from build123d import *

# Parameters (mm, degrees)
SKETCH3_W           = 76.2
SKETCH3_H           = 76.2
BOSS_EXTRUDE2_DEPTH = 101.6
SKETCH4_R           = 6.35
CUT_EXTRUDE2_DEPTH  = 73.914
SKETCH5_R           = 25.4
CUT_EXTRUDE3_DEPTH  = 113.538
SKETCH7_R           = 6.35
CUT_EXTRUDE4_DEPTH  = 18.034


with BuildPart() as part:
    # Sketch3 → Boss-Extrude2 (new body)
    with BuildSketch(Plane(origin=(0, 0, 0), x_dir=(1, 0, 0), z_dir=(0, 1, 0))):
        with Locations((38.1, 38.1)):
            Rectangle(SKETCH3_W, SKETCH3_H)
    extrude(amount=BOSS_EXTRUDE2_DEPTH)

    # Sketch4 → Cut-Extrude2 (cut)
    with BuildSketch(Plane.XY):
        with Locations((38.1, 50.8)):
            Circle(SKETCH4_R)
    extrude(amount=-CUT_EXTRUDE2_DEPTH, mode=Mode.SUBTRACT)

    # Sketch5 → Cut-Extrude3 (cut)
    with BuildSketch(Plane(origin=(0, 101.6, 0), x_dir=(1, 0, 0), z_dir=(0, 1, 0))):
        with Locations(Location((38.1, 38.1, 0), (0, 0, 270))):
            Circle(SKETCH5_R)
    extrude(amount=-CUT_EXTRUDE3_DEPTH, mode=Mode.SUBTRACT)

    # Sketch7 → Cut-Extrude4 (cut)
    with BuildSketch(Plane(origin=(0, 0, -76.2), x_dir=(-1, 0, 0), z_dir=(0, 0, -1))):
        with Locations(Location((-38.1, 50.8, 0), (0, 0, 180))):
            Circle(SKETCH7_R)
    extrude(amount=-CUT_EXTRUDE4_DEPTH, mode=Mode.SUBTRACT)


solid = part.part
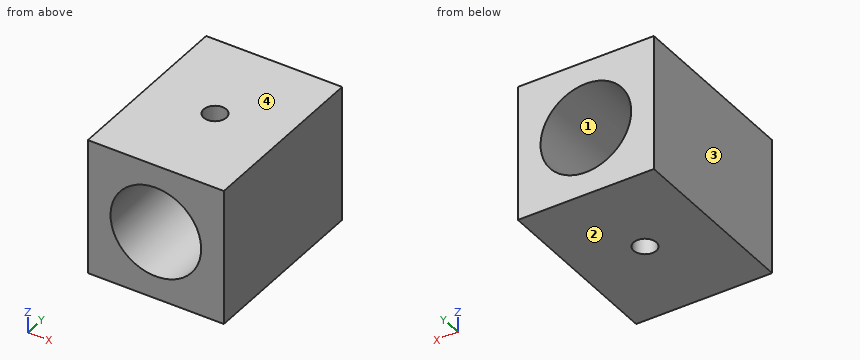
Geometry check sheet. Reference: the model listing, model coordinates, mm. Face numbers are marked on the shaded views. Give positions to 0.01 mm unless a question says otherwise; leave off trailing zeros. Write each loop counter-clockwise with the first axis right and the second up, starting at its lowest first coordinate (ties: lowest second). Pieces come first, ordered by that corner, then holes. Notation, with made-up numbers: M -8,65.5 L 33,65.5 A26 cw 33,86.5 Z; hole C -34.75,-33.75 d8. An arc over 180 degrees is marked long. Answer as CSV lines item,"result". Start each with the question number.
Q1. Section check B-B, the plane y = 50.8. Record the cut outline in (x, z).
Q2. Release check for a two-part mould opening along Z. For the marked faces 1, 2, 3 and 4 record: pulls with the +Z half, pulls with the -Z half, needs draft (parallel to the pull), parting line crosses it, or undercut.
Q3. Material ranges on L1, parallel to X at y = 37, z = -38.1; L2, parallel to Y at x = 38.1, z = -66; L3, parallel to Z at x = 38, y = 21, recorded low to high.
Q4. Section check D-D, the plane x = 51.5. Record the cut outline in (y, z).
Q5. Section check C-C, the plane x = 38.1. Record the cut outline in (y, z), then the cut area to 3 significant figures.
Q6. Section check A-A, the plane z = -38.1. Record the cut outline in (x, y), then the cut area to 3 significant figures.
Geometry says:
1,outline,"M 0,-76.2 L 31.75,-76.2 L 31.75,-62.69 A25.4 cw 31.75,-13.51 L 31.75,0 L 0,0 Z; M 44.45,-76.2 L 76.2,-76.2 L 76.2,0 L 44.45,0 L 44.45,-13.51 A25.4 cw 44.45,-62.69 Z"
2,face 1,"undercut"
2,face 2,"pulls with the -Z half"
2,face 3,"needs draft"
2,face 4,"pulls with the +Z half"
3,L1,"0 to 12.7, 63.5 to 76.2"
3,L2,"0 to 44.45, 57.15 to 101.6"
3,L3,"-76.2 to -63.5, -12.7 to 0"
4,outline,"M 0,-76.2 L 101.6,-76.2 L 101.6,-59.68 L 0,-59.68 Z; M 0,-16.52 L 101.6,-16.52 L 101.6,0 L 0,0 Z"
5,outline,"M 0,-76.2 L 44.45,-76.2 L 44.45,-63.5 L 0,-63.5 Z; M 0,-12.7 L 44.45,-12.7 L 44.45,0 L 0,0 Z; M 57.15,-76.2 L 101.6,-76.2 L 101.6,-63.5 L 57.15,-63.5 Z; M 57.15,-12.7 L 101.6,-12.7 L 101.6,0 L 57.15,0 Z"
5,area,"2,260 mm^2"
6,outline,"M 0,0 L 12.7,0 L 12.7,101.6 L 0,101.6 Z; M 63.5,0 L 76.2,0 L 76.2,101.6 L 63.5,101.6 Z"
6,area,"2,580 mm^2"
